Work out the finished part from the listing and answer in its coordinate system (mm). Give positions to 0.01 mm unless a question says otherwise; leave off trailing zeros. Loops run counter-clockwise (first coordinate to the right, second up) from the corner with the lowest first, then second, coordinate; pieces in that order, holes last.
```python
from build123d import *

# Parameters (mm, degrees)
SKETCH1_R           = 6.35
BOSS_EXTRUDE1_DEPTH = 152.4
CUT_EXTRUDE1_DEPTH  = 18.034
CUT_EXTRUDE2_DEPTH  = 38.1


with BuildPart() as part:
    # Sketch1 → Boss-Extrude1 (new body)
    with BuildSketch(Plane.XY):
        with Locations(Location((0, 0, 0), (0, 0, 180))):
            Circle(SKETCH1_R)
    extrude(amount=BOSS_EXTRUDE1_DEPTH)

    # Sketch2 → Cut-Extrude1 (cut)
    with BuildSketch(Plane(origin=(0, 0, 12.7), x_dir=(-1, 0, 0), z_dir=(0, 0, -1))):
        Polygon((1.571433325, 4.7625), (-0.016066675, 4.7625), (-1.603566675, 4.7625), (-1.603566675, 7.9375), (1.571433325, 7.9375), align=None)
    extrude(amount=-CUT_EXTRUDE1_DEPTH, mode=Mode.SUBTRACT)

    # Sketch3 → Cut-Extrude2 (cut)
    with BuildSketch(Plane.XY.offset(146.05)):
        Polygon((0, 4.7625), (1.5875, 4.7625), (1.5875, 7.9375), (-1.5875, 7.9375), (-1.5875, 4.7625), align=None)
    extrude(amount=-CUT_EXTRUDE2_DEPTH, mode=Mode.SUBTRACT)


solid = part.part
```
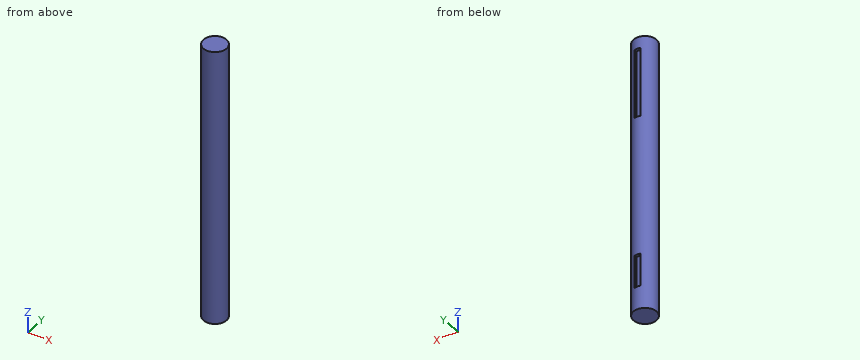
Q1. Given pin 1 (1.1 mm diameter, centred on y = 5.5, z = 136, fed in from -X); pin 2 (3.5 mm diameter, centred on x = 0, z = 18.5, fed in from +Y); pin 3 (1.5 mm diameter, centred on y = 5, z = 23.5, fed in from -X), each flat-ended and moving along its own axis, determine where each tip first touches the part or whether it passes through.
Q2. Section A-A on x = 0 is taken. Give the vertices of the cut face in (y, z), plus the area to 3 significant figures.
Q3. Section D-D on z = 127 is taken. Give the vertices of the cut face in (x, y).
Q4. Section B-B on z = 9 is taken. Give the vertices of the cut face in (x, y), plus the area to 3 significant figures.
Q5. Section C-C on y = 3.25 is taken. Give the vertices of the cut face in (x, z).
Q6. Consider line 1 along Y through (x, z) = (0, 123); line 2 along X through (y, z) = (5.75, 135); line 3 along Y through (x, z) = (4.25, 53.5). Determine where each line is inside the solid, lowest interval first.
Check result:
1. pin 1: stops at x = -3.98
1. pin 2: stops at y = 6.15
1. pin 3: stops at x = -4.72
2. outline: (-6.35, 0) - (6.35, 0) - (6.35, 12.7) - (4.76, 12.7) - (4.76, 30.73) - (6.35, 30.73) - (6.35, 107.95) - (4.76, 107.95) - (4.76, 146.05) - (6.35, 146.05) - (6.35, 152.4) - (-6.35, 152.4) - close
2. area: 1,850 mm2
3. outline: (-1.59, 4.76) - (-1.59, 6.15) arc R6.35 ccw (long way) to (1.59, 6.15) - (1.59, 4.76) - close
4. outline: circle Ø12.7 at (0, 0)
4. area: 127 mm2
5. outline: (-5.46, 0) - (5.46, 0) - (5.46, 152.4) - (-5.46, 152.4) - close
6. line 1: y = -6.35 to 4.76
6. line 2: x = -2.69 to -1.59, 1.59 to 2.69
6. line 3: y = -4.72 to 4.72
